Source: CAD feature listing. Evaluate the final solid. Frame: model axes, mm. A direction names the side the tool comes from. Give positions to 0.01 mm unless a question says otherwise; leave off trailing zeros. Order: outer loops, then holes, each group sorted by start corner. A loop starts at its lowest first (then second) coordinate and runs counter-clockwise, first axis right, second up.
1) Section D-D, the plane z = -87. Return loops of the section in (x, y) (3 decimals).
2) Section B-B, the plane z = -57. Return loops of the section in (x, y) (1 decimal), plus the area to 3 significant figures.
3) Section C-C, the plane y = -0.75. Return loops of the section in (x, z).
4) Material intervals for line 1 (Y direction, x = 43, z = -63.5) (3 decimals); line 2 (X direction, y = -1, z = -63); line 3 (Z direction, x = 69, y = 3.25), sorted ascending.
5) Access query for faces 4 (the face through (31, 3.175, -18)), 5 (the face through (0, 0, -47)), 6 (the face through (31, 3.175, -79)). Directions: +Z, -Z, +X, -X, +Y, -Y. A direction counts if a zero-diameter tool reaches every point of the face in a straight line with its end or side. Return the directions, or none.
6) First-contact query: P1, Ø1.9, axis at x = -14.74, z = -48.73, coming from the +Y side; P2, Ø2, axis at y = 3.5, z = -43, coming from the -X side; P3, Ø4, axis at x = 61, z = -75.5, coming from the +Y side (3 decimals); P4, Ø0.5, axis at x = 42.5, y = 3.5, coming from the +Z side. Flat tips, straight axial feed; report the tip coordinate or a pass-through.
7) Draft query along X for faces 1 (the face through (63.5, 0, -47)), 2 (the face through (31, 0, 0)), 3 (the face through (77.534, 3.958, -50.071)). Return one class per face: released by +X, released by -X, zero draft, split by the parting line, or undercut.
```python
from build123d import *

# Parameters (mm, degrees)
SKETCH1_W           = 63.5
SKETCH1_H           = 95.25
BOSS_EXTRUDE1_DEPTH = 3.175
SKETCH2_R           = 1.5875
BOSS_EXTRUDE2_DEPTH = 1.5875


with BuildPart() as part:
    # Sketch1 → Boss-Extrude1 (new body, symmetric)
    with BuildSketch(Plane(origin=(0, 0, 0), x_dir=(1, 0, 0), z_dir=(0, 1, 0))):
        with Locations((31.75, 47.625)):
            Rectangle(SKETCH1_W, SKETCH1_H)
    extrude(amount=BOSS_EXTRUDE1_DEPTH, both=True)

    # Sketch2 → Boss-Extrude2 (add)
    with BuildSketch(Plane(origin=(0, 3.175, 0), x_dir=(1, 0, 0), z_dir=(0, 1, 0))):
        with BuildLine():
            Line((-19.831384914, 36.032499706), (81.768615086, 36.032499706))
            ThreePointArc((81.768615086, 36.032499706), (87.029127328, 48.732499706), (81.768615086, 61.432499706))
            Line((81.768615086, 61.432499706), (-19.831384914, 61.432499706))
            ThreePointArc((-19.831384914, 61.432499706), (-25.091897156, 48.732499706), (-19.831384914, 36.032499706))
        make_face()
        with Locations((-14.743661756, 48.732499706)):
            Circle(SKETCH2_R, mode=Mode.SUBTRACT)
        with Locations((76.680891929, 48.732499706)):
            Circle(SKETCH2_R, mode=Mode.SUBTRACT)
    extrude(amount=BOSS_EXTRUDE2_DEPTH)


solid = part.part
```
From the geometry:
1. outline: (0, -3.175) - (63.5, -3.175) - (63.5, 3.175) - (0, 3.175) - close
2. outline: (-23.1, 3.2) - (0, 3.2) - (0, -3.2) - (63.5, -3.2) - (63.5, 3.2) - (85, 3.2) - (85, 4.8) - (-23.1, 4.8) - close
2. area: 575 mm2
3. outline: (0, -95.25) - (63.5, -95.25) - (63.5, 0) - (0, 0) - close
4. line 1: y = -3.175 to 3.175
4. line 2: x = 0 to 63.5
4. line 3: z = -61.43 to -36.03
5. face 4: +Z, +X, -X, +Y
5. face 5: +Z, -Z, -X, -Y
5. face 6: -Z, +X, -X, +Y
6. P1: passes through
6. P2: stops at x = -24.46
6. P3: stops at y = 3.175
6. P4: stops at z = -36.03
7. face 1: released by +X
7. face 2: zero draft
7. face 3: undercut
